Work out the finished part from the listing and answer in its coordinate system (mm). Round coordinates to 2 decimals unless told otherwise and drop trailing zeros. Order: outer loops, then holes, each group sorted by start corner. A loop starts at its lowest first (then second) coordinate and runs counter-clockwise, first axis right, second up. Notation, with made-up numbers: M 0,26.25 L 48,26.25 A15 ccw 48,51.25 Z; hole C -1,9.5 d7. An arc over 180 degrees is marked long. Return JSON: item names as keys, results as strings.
from build123d import *

# Parameters (mm, degrees)
CYLINDER022_R          = 5
CYLINDER022_DEPTH      = 9
CYLINDER022_ROLL_ANGLE = 90
BOX030_W               = 8
BOX030_H               = 9
BOX030_DEPTH           = 16
CYLINDER021_R          = 8
CYLINDER021_DEPTH      = 9
CYLINDER021_ROLL_ANGLE = 90


with BuildPart() as zylinder008:
    # Cylinder022 → Cylinder022 (new body)
    with BuildSketch(Plane.XY):
        Circle(CYLINDER022_R)
    extrude(amount=CYLINDER022_DEPTH)


with BuildPart() as zylinder008_1:
    # Cylinder022 roll: moved
    add(zylinder008.part.rotate(Axis((0, 0, 0), (1, 0, 0)), CYLINDER022_ROLL_ANGLE))


with BuildPart() as zylinder008_2:
    # Cylinder022 placement: moved
    add(zylinder008_1.part.moved(Location((8, 9, 8))))


with BuildPart() as obj1:
    # Box030 → Box030 (new body)
    with BuildSketch(Plane.XY):
        with Locations((4, 4.5)):
            Rectangle(BOX030_W, BOX030_H)
    extrude(amount=BOX030_DEPTH)


with BuildPart() as obj2:
    # Cylinder021 → Cylinder021 (new body)
    with BuildSketch(Plane.XY):
        Circle(CYLINDER021_R)
    extrude(amount=CYLINDER021_DEPTH)


with BuildPart() as obj2_1:
    # Cylinder021 roll: moved
    add(obj2.part.rotate(Axis((0, 0, 0), (1, 0, 0)), CYLINDER021_ROLL_ANGLE))


with BuildPart() as obj2_2:
    # Cylinder021 placement: moved
    add(obj2_1.part.moved(Location((8, 9, 8))))

    # Fusion015: union obj1
    add(obj1.part)

    # Cut020: cut Zylinder008
    add(zylinder008_2.part, mode=Mode.SUBTRACT)


with BuildPart() as obj2_3:
    # Cut020 placement: moved
    add(obj2_2.part.moved(Location((160, 10, 20))))


solid = obj2_3.part
Item 1: Find section C-C (y = 15.5). Determine the outline of the cut face in (x, z), plus the area to 3 significant figures.
Output:
{"outline": "M 160,20 L 168,20 A8 ccw 168,36 L 160,36 Z; hole C 168,28 d10", "area": "150 mm^2"}
Item 2: Each of these flat-tipped pins is pushed along its axis until it touches: pin 1 (1.5 mm diameter, centred on x = 168, z = 32, fed in from +Y); pin 2 (3 mm diameter, centred on y = 16, z = 31, fed in from +X); pin 3 (4 mm diameter, centred on y = 16.5, z = 26.5, fed in from +X). Where does it stop, or does it pass through?
Output:
{"pin 1": "passes through", "pin 2": "stops at x = 175.86", "pin 3": "stops at x = 176"}
Item 3: Consider line 1 along Z through (x, y) = (168, 17); line 2 along X through (y, z) = (11, 30.5); line 3 along X through (y, z) = (17.75, 28.75). Determine where each line is inside the solid, lowest interval first. Write a range as [from, to].
Output:
{"line 1": "z = [20, 23], [33, 36]", "line 2": "x = [160, 163.67], [172.33, 175.6]", "line 3": "x = [160, 163.06], [172.94, 175.96]"}
Item 4: Find section B-B (x = 165). Determine the outline of the cut face in (y, z), plus the area to 3 significant figures.
Output:
{"outline": "M 10,20 L 19,20 L 19,24 L 10,24 Z; M 10,32 L 19,32 L 19,36 L 10,36 Z", "area": "72.0 mm^2"}
Item 5: The mould has two halves that part along Z. Classify faces 1 (the flat face through (162.6, 10, 27.9)), 2 (the cylindrical face through (176, 15, 28)), 3 (the cylindrical face through (164, 15, 25)): pulls with the +Z half, pulls with the -Z half, needs draft (parallel to the pull), parting line crosses it, or undercut.
Output:
{"face 1": "needs draft", "face 2": "parting line crosses it", "face 3": "undercut"}
Item 6: Find section D-D (x = 174.25). Determine the outline of the cut face in (y, z), plus the area to 3 significant figures.
Output:
{"outline": "M 10,23.01 L 19,23.01 L 19,32.99 L 10,32.99 Z", "area": "89.9 mm^2"}
Item 7: Find section A-A (z = 28). Determine the outline of the cut face in (x, y).
Output:
{"outline": "M 160,10 L 163,10 L 163,19 L 160,19 Z; M 173,10 L 176,10 L 176,19 L 173,19 Z"}
